The model under review builds one solid part; all positions refer to its coordinate system, in mm. A direction names the side the tool comes from. Coordinates: 2 decimals unless noted, no trailing zeros. Loops run counter-clockwise (first coordinate to the right, second up) from the corner with the lowest first, then second, coordinate; pieces in that order, holes last. Notation, with made-up numbers: M 31.5,68 L 54.5,68 A21 cw 54.5,105 Z; hole C -35.75,83.25 d11. An arc over 180 degrees is marked long. Write item = value, one per line. Start each with the question number.
Q1. Mouldability with a two-part tool opening along Z and no side actions: class faces 3 (the face through (22, 2, 0)), 4 (the face through (61.586, 2.465, 9.792)), 5 (the face through (80, 2, 15)) as released by +Z, released by -Z, zero draft, split by the parting line, or undercut.
Q2. We need section C-C on x = -22.65. Give the boundary of the cut face in (y, z), and give its area (3 significant figures).
Q3. Wall thickness on probe 1 along X at (y, z) = (1.6, 17.5); probe 2 along X at (y, z) = (1.15, 33.5); probe 3 along X at (y, z) = (0.4, 46): over which ranges is each line inside the solid? List them lowest first.
Q4. We need section A-A on z = 20. Give the boundary of the cut face in (x, y).
Q5. We need section B-B on y = 3.2. Count the separate pieces of the cut face and the enclosed holes in it, and give its area (3 significant figures).
Q6. Clearance check with flat-ended pins moving along their axes: pin 1 Ø2 at (x, z) = (-22.65, 17.5) entering from -Y; pin 2 Ø3 at (x, y) = (61, 2.5) entering from +Z; pin 3 Ø3.5 at (x, z) = (-2.65, 33.5) entering from -Y; pin 4 Ø2.5 at (y, z) = (3, 45.5) entering from +X. State where each tip first meets the part, or that it passes through.
Q7. For faces 1 (the face through (43, 2, 30)), 2 (the face through (61.586, 2.465, 19.792)), list the 3-axis set-ups (+Z, -Z, +X, -X, +Y, -Y) from which the entire face can be reached by the end or side of a thin tool; tool diameter is ignored.
Q8. We need section D-D on x = 27. Give the boundary of the cut face in (y, z), and give its area (3 significant figures).
from build123d import *

# Parameters (mm, degrees)
SKETCH1_R           = 1.4
SKETCH1_R_2         = 1.6
SKETCH1_W           = 8
SKETCH1_H           = 24
BOSS_EXTRUDE1_DEPTH = 5


with BuildPart() as part:
    # Sketch1 → Boss-Extrude1 (new body)
    # profile 1 of 3: a face of its own
    with BuildSketch(Plane(origin=(0, 0, 0), x_dir=(1, 0, 0), z_dir=(0, 1, 0))):
        Polygon((0, -30), (0, 0), (-37.9, 0), (-37.9, -35), (-37.9, -54), (0, -54), align=None)
        with Locations(Location((-22.65, -33.5, 0), (0, 0, 270))):
            Circle(SKETCH1_R, mode=Mode.SUBTRACT)
        with Locations(Location((-2.65, -33.5, 0), (0, 0, 270))):
            Circle(SKETCH1_R, mode=Mode.SUBTRACT)
        with Locations(Location((-22.65, -17.5, 0), (0, 0, 270))):
            Circle(SKETCH1_R, mode=Mode.SUBTRACT)
        with Locations(Location((-2.65, -17.5, 0), (0, 0, 270))):
            Circle(SKETCH1_R, mode=Mode.SUBTRACT)
    # profile 2 of 3: a face of its own
    with BuildSketch(Plane(origin=(0, 0, 0), x_dir=(1, 0, 0), z_dir=(0, 1, 0))):
        Polygon((80, 0), (0, 0), (0, -30), (8, -30), (80, -30), align=None)
        with Locations(Location((30, -20, 0), (0, 0, 270))):
            Circle(SKETCH1_R_2, mode=Mode.SUBTRACT)
        with Locations(Location((60, -20, 0), (0, 0, 270))):
            Circle(SKETCH1_R_2, mode=Mode.SUBTRACT)
        with Locations(Location((30, -10, 0), (0, 0, 270))):
            Circle(SKETCH1_R_2, mode=Mode.SUBTRACT)
        with Locations(Location((60, -10, 0), (0, 0, 270))):
            Circle(SKETCH1_R_2, mode=Mode.SUBTRACT)
    # profile 3 of 3: a face of its own
    with BuildSketch(Plane(origin=(0, 0, 0), x_dir=(1, 0, 0), z_dir=(0, 1, 0))):
        with Locations((4, -42)):
            Rectangle(SKETCH1_W, SKETCH1_H)
    extrude(amount=BOSS_EXTRUDE1_DEPTH)


solid = part.part
Returned:
q1.face_3 = released by -Z
q1.face_4 = undercut
q1.face_5 = zero draft
q2.outline = M 0,0 L 5,0 L 5,16.1 L 0,16.1 Z; M 0,18.9 L 5,18.9 L 5,32.1 L 0,32.1 Z; M 0,34.9 L 5,34.9 L 5,54 L 0,54 Z
q2.area = 242 mm^2
q3.probe_1 = -37.9 to -24.05, -21.25 to -4.05, -1.25 to 80
q3.probe_2 = -37.9 to -24.05, -21.25 to -4.05, -1.25 to 8
q3.probe_3 = -37.9 to 8
q4.outline = M -37.9,0 L 28.4,0 L 28.4,5 L -37.9,5 Z; M 31.6,0 L 58.4,0 L 58.4,5 L 31.6,5 Z; M 61.6,0 L 80,0 L 80,5 L 61.6,5 Z
q5.separate_pieces = 1
q5.enclosed_holes = 8
q5.area = 4,580 mm^2
q6.pin_1 = through
q6.pin_2 = 30
q6.pin_3 = 0
q6.pin_4 = 8
q7.face_1 = +Z, +X, +Y, -Y
q7.face_2 = +Y, -Y
q8.outline = M 0,0 L 5,0 L 5,30 L 0,30 Z
q8.area = 150 mm^2
